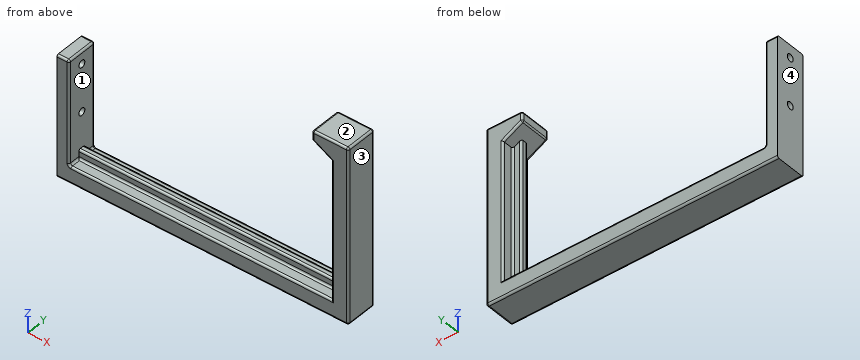
```python
from build123d import *

# Parameters (mm, degrees)
F1_DEPTH = 6.5
F2_R     = 1.5
F3_DEPTH = 25
F5_DEPTH = 1.5
F6_R     = 0.8


with BuildPart() as f1:
    # F0 (on Front) → F1 (new body, symmetric)
    with BuildSketch(Plane.XZ):
        Polygon((-72.959999821, 50), (-72.959999821, 0), (47.040000179, 0), (47.040000179, 72.3599994255), (32.040000179, 72.3599994255), (32.040000179, 68.3599994255), (40.040000179, 64), (40.040000179, 7), (-67.959999821, 7), (-67.959999821, 50), align=None)
    extrude(amount=F1_DEPTH, both=True)

    # F2 (on face) → F3 (cut)
    with BuildSketch(Plane(origin=(-72.959999821, 0, 0), x_dir=(0, -1, 0), z_dir=(-1, 0, 0))):
        with Locations((0, 25.1972917467)):
            Circle(F2_R)
        with Locations((0, 44.7687469423)):
            Circle(F2_R)
    extrude(amount=-F3_DEPTH, mode=Mode.SUBTRACT)

    # F4 (on Front) → F5 (join, symmetric)
    with BuildSketch(Plane.XZ):
        Polygon((-71.5028345585, 10.6206643313), (-71.5028345585, 7.5510139577), (-71.5028345585, 5.6206643313), (41.4378745708, 5.6206643313), (41.4378745708, 70.8550155432), (36.4378745708, 70.8550155432), (36.4378745708, 10.6206643313), align=None)
    extrude(amount=F5_DEPTH, both=True)

    # F6
    f6_edges = [f1.edges().sort_by_distance(p)[0] for p in [
        (-67.96, -6.5, 28.5),
        (-67.96, 0, 50),
        (-70.46, 6.5, 50),
        (-70.46, -6.5, 50),
        (-67.96, 6.5, 28.5),
        (-13.96, 6.5, 7),
        (-15.761063, 1.5, 10.620664),
        (-15.761063, -1.5, 10.620664),
        (-13.96, -6.5, 7),
        (40.04, -6.5, 35.5),
        (36.437875, -1.5, 38.291911),
        (36.437875, 1.5, 38.291911),
        (40.04, 6.5, 35.5),
        (47.04, 6.5, 36.18),
        (-12.96, 6.5, 0),
        (-12.96, -6.5, 0),
        (47.04, -6.5, 36.18),
        (47.04, 0, 72.359999),
        (32.04, 0, 72.359999),
        (39.54, 6.5, 72.359999),
        (39.54, -6.5, 72.359999),
        (32.04, 0, 68.359999),
        (36.04, -6.5, 66.18),
        (36.04, 6.5, 66.18),
        (40.04, 1.5, 35.5),
        (40.04, -1.5, 35.5),
        (32.04, -6.5, 70.359999),
        (32.04, 6.5, 70.359999),
        (-13.96, -1.5, 7),
        (-13.96, 1.5, 7),
        (47.04, 0, 0),
        (-67.96, -4, 7),
        (-67.96, 4, 7),
    ]]
    fillet(f6_edges, radius=F6_R)


solid = f1.part
```
Model file for the job. Use its own axes, mm. Face numbers are marked on the shaded views. Round coordinates to 2 decimals unless told otherwise and drop trailing zeros. Loops run counter-clockwise (first coordinate to the right, second up) from the corner with the lowest first, then second, coordinate; pieces in that order, holes last. Notation, with made-up numbers: M -35,33.25 L 13,33.25 A23 cw 13,59.25 Z; hole C -1.75,59 d7. An arc over 180 degrees is marked long. Put each result on its own line as item: value. Start each with the question number.
Item 1: Drill centre lines: line 1 along Z through (x, y) = (-70.2, 0); line 2 along X through (y, z) = (4.5, 26); line 3 along X through (y, z) = (-2.25, 51.5). Where is each one in solid material? Low to high.
Item 2: Cut at A-A (z = 42). List the corners of the cut face in (x, y).
Item 3: Mould opens along X. For the marked faces 1, 2, 3 and 4 say: released by +X, released by -X, zero draft, split by the parting line, or undercut.
Item 4: Drop flat-ended pins along their axis: P1, Ø6, axis at x = 9.5, z = 10.5, coming from the -Y side; P2, Ø3.5, axis at x = -25.5, y = 4.5, coming from the +Z side; P3, Ø3, axis at y = -0.5, z = 70.5, coming from the -X side. Give the stop position or say it passes through.
Item 5: Cut at B-B (x = -60). List the corners of the cut face in (y, z), then the cut area to 3 significant figures.
Item 6: Cut at C-C (y = -4.5). List the corners of the cut face in (x, z).
Answer block:
1. line 1: 0 to 23.7, 26.7 to 43.27, 46.27 to 50
1. line 2: -72.96 to -67.96, 40.04 to 47.04
1. line 3: 40.04 to 47.04
2. outline: M -72.96,-6.5 L -68.76,-6.5 A0.8 ccw -67.96,-5.7 L -67.96,5.7 A0.8 ccw -68.76,6.5 L -72.96,6.5 Z; M 36.44,-0.7 A0.8 ccw 37.24,-1.5 L 39.24,-1.5 A0.8 cw 40.04,-2.3 L 40.04,-5.7 A0.8 ccw 40.84,-6.5 L 46.24,-6.5 A0.8 ccw 47.04,-5.7 L 47.04,5.7 A0.8 ccw 46.24,6.5 L 40.84,6.5 A0.8 ccw 40.04,5.7 L 40.04,2.3 A0.8 cw 39.24,1.5 L 37.24,1.5 A0.8 ccw 36.44,0.7 Z
3. face 1: undercut
3. face 2: zero draft
3. face 3: released by +X
3. face 4: released by -X
4. P1: y = -1.56
4. P2: z = 7
4. P3: x = 32.04
5. outline: M -6.5,0.8 A0.8 ccw -5.7,0 L 5.7,0 A0.8 ccw 6.5,0.8 L 6.5,6.2 A0.8 ccw 5.7,7 L 2.3,7 A0.8 cw 1.5,7.8 L 1.5,9.82 A0.8 ccw 0.7,10.62 L -0.7,10.62 A0.8 ccw -1.5,9.82 L -1.5,7.8 A0.8 cw -2.3,7 L -5.7,7 A0.8 ccw -6.5,6.2 Z
5. area: 101 mm2
6. outline: M -72.96,0 L 46.24,0 A0.8 ccw 47.04,0.8 L 47.04,71.56 A0.8 ccw 46.24,72.36 L 32.84,72.36 A0.8 ccw 32.04,71.56 L 32.04,68.84 A0.8 ccw 32.46,68.13 L 40.04,64 L 40.04,7 L -67.16,7 A0.8 cw -67.96,7.8 L -67.96,49.2 A0.8 ccw -68.76,50 L -72.96,50 Z
